Design review of the part built by this model. Coordinates are the model's own, in mm. A direction names the side the tool comes from. Coordinates: 2 decimals unless noted, no trailing zeros. Loops run counter-clockwise (first coordinate to the right, second up) from the corner with the lowest first, then second, coordinate; pieces in that order, holes last. Notation, with made-up numbers: (14, -3) -> (34, -3) arc R36 cw to (34, 36) -> close; hole circle Ø3 at (83.5, 62). An arc over 180 degrees is marked (long way). Use a Markdown table: item, result. Add a question column.
Q1. Take a section at A-A on y = 28. Write out the cut boundary in (x, z), plus the area to 3 significant figures.
Q2. Draft analysis for pull direction X (two halves, no side actions). For faces 3 (the face through (-107.984, 12, -49)), 4 (the face through (-17, 12, 39.984)), 5 (the face through (24, 5, -92)), state which applies: pulls with the +X half, pulls with the -X half, needs draft (parallel to the pull), parting line crosses it, or undercut.
Q3. Take a section at C-C on z = 25. Write out the cut boundary in (x, y), plus the area to 3 significant figures.
Q4. For probe 1 along Z at (x, y) = (-18.5, 8); probe 2 along Y at (x, z) = (-91, -137.5); probe 3 along Z at (x, y) = (69, 11), list the stretches that pass through material, from the lowest coordinate up.
Q5. Clearance check with flat-ended pins moving along their axes: pin 1 Ø10 at (x, y) = (23.5, 31) entering from +Z; pin 2 Ø8 at (y, z) = (43.5, -14) entering from +X; pin 3 Ø3 at (y, z) = (34, -48.5) entering from -X. State where each tip first meets the part, or that it passes through.
Q6. Take a section at B-B on z = -148.5. Write out the cut boundary in (x, y), plus the area to 3 significant figures.
Q7. For faces 1 (the face through (-42.558, 6.504, -135.362)), 2 (the face through (-88, 12, -150)), list the 3-axis set-ups (+Z, -Z, +X, -X, +Y, -Y) from which the entire face can be reached by the end or side of a thin tool; tool diameter is ignored.
from build123d import *

# Parameters (mm, degrees)
F1_DEPTH = 50
F2_DEPTH = 25
F4_DEPTH = 5
F5_R     = 5


with BuildPart() as f1:
    # F0 (on Front) → F1 (new body)
    with BuildSketch(Plane.XZ):
        with BuildLine():
            Line((-14.1471050896, 14.137164411), (-81.6470713128, -53.4102650408))
            ThreePointArc((-81.6470713128, -53.4102650408), (-81.4172585272, -82.8327909518), (-52.1131197981, -80.1860385553))
            Line((-52.1131197981, -80.1860385553), (14.1195211891, -14.1647139537))
            ThreePointArc((14.1195211891, -14.1647139537), (14.1509459034, 14.133319852), (-14.1471050896, 14.137164411))
        make_face()
        with BuildLine():
            ThreePointArc((-7.0735915388, 7.0685431839), (7.0736510846, 7.068483595), (7.0633719628, -7.0787552942))
            Line((7.0633719628, -7.0787552942), (-62.1351958298, -76.1269429069))
            ThreePointArc((-62.1351958298, -76.1269429069), (-75.7541474378, -74.3104584003), (-74.7048583437, -60.6110258843))
            Line((-74.7048583437, -60.6110258843), (-7.0735915388, 7.0685431839))
        make_face(mode=Mode.SUBTRACT)
    extrude(amount=-F1_DEPTH)

    # F0 (on Front) → F2 (join)
    with BuildSketch(Plane.XZ):
        with BuildLine():
            Line((102.0160578582, -0.0157058509), (62.0160578582, 39.9842941491))
            Line((62.0160578582, 39.9842941491), (-97.9839421418, 39.9842941491))
            ThreePointArc((-97.9839421418, 39.9842941491), (-105.0550099537, 37.055361961), (-107.9839421418, 29.9842941491))
            Line((-107.9839421418, 29.9842941491), (-107.9839421418, -130.0157058509))
            Line((-107.9839421418, -130.0157058509), (-67.9839421418, -170.0157058509))
            Line((-67.9839421418, -170.0157058509), (92.0160578582, -170.0157058509))
            ThreePointArc((92.0160578582, -170.0157058509), (99.0871256701, -167.0867736627), (102.0160578582, -160.0157058509))
            Line((102.0160578582, -160.0157058509), (102.0160578582, -0.0157058509))
        make_face()
        with BuildLine():
            ThreePointArc((93.0160578582, -91.0157058509), (90.0871256701, -98.0867736627), (83.0160578582, -101.0157058509))
            Line((83.0160578582, -101.0157058509), (57.0160578582, -101.0157058509))
            ThreePointArc((57.0160578582, -101.0157058509), (40.0454951097, -108.0451431024), (33.0160578582, -125.0157058509))
            Line((33.0160578582, -125.0157058509), (33.0160578582, -151.0157058509))
            ThreePointArc((33.0160578582, -151.0157058509), (30.0871256701, -158.0867736627), (23.0160578582, -161.0157058509))
            Line((23.0160578582, -161.0157058509), (-33.9839421418, -161.0157058509))
            ThreePointArc((-33.9839421418, -161.0157058509), (-41.0550099537, -158.0867736627), (-43.9839421418, -151.0157058509))
            Line((-43.9839421418, -151.0157058509), (-43.9839421418, -119.263347337))
            ThreePointArc((-43.9839421418, -119.263347337), (-41.9657763558, -113.2392023702), (-36.7258776257, -109.6466020559))
            ThreePointArc((-36.7258776257, -109.6466020559), (12.6262309135, -80.6258789061), (41.6469540632, -31.273770367))
            ThreePointArc((41.6469540632, -31.273770367), (45.2395543775, -26.0338716369), (51.2636993443, -24.0157058509))
            Line((51.2636993443, -24.0157058509), (83.0160578582, -24.0157058509))
            ThreePointArc((83.0160578582, -24.0157058509), (90.0871256701, -26.944638039), (93.0160578582, -34.0157058509))
            Line((93.0160578582, -34.0157058509), (93.0160578582, -91.0157058509))
        make_face(mode=Mode.SUBTRACT)
        with BuildLine():
            ThreePointArc((-52.1131197981, -80.1860385553), (-81.4172585272, -82.8327909518), (-81.6470713128, -53.4102650408))
            Line((-81.6470713128, -53.4102650408), (-14.1471050896, 14.137164411))
            ThreePointArc((-14.1471050896, 14.137164411), (14.1509459034, 14.133319852), (14.1195211891, -14.1647139537))
            Line((14.1195211891, -14.1647139537), (-52.1131197981, -80.1860385553))
        make_face(mode=Mode.SUBTRACT)
    extrude(amount=-F2_DEPTH)

    # F3 (on face) → F4 (join)
    with BuildSketch(Plane.XZ):
        with BuildLine():
            ThreePointArc((51.2636993443, -24.0157058509), (45.2395543775, -26.0338716369), (41.6469540632, -31.273770367))
            ThreePointArc((41.6469540632, -31.273770367), (12.6262309135, -80.6258789061), (-36.7258776257, -109.6466020559))
            ThreePointArc((-36.7258776257, -109.6466020559), (-41.9657763558, -113.2392023702), (-43.9839421418, -119.263347337))
            Line((-43.9839421418, -119.263347337), (-43.9839421418, -151.0157058509))
            ThreePointArc((-43.9839421418, -151.0157058509), (-41.0550099537, -158.0867736627), (-33.9839421418, -161.0157058509))
            Line((-33.9839421418, -161.0157058509), (23.0160578582, -161.0157058509))
            ThreePointArc((23.0160578582, -161.0157058509), (30.0871256701, -158.0867736627), (33.0160578582, -151.0157058509))
            Line((33.0160578582, -151.0157058509), (33.0160578582, -125.0157058509))
            ThreePointArc((33.0160578582, -125.0157058509), (40.0454951097, -108.0451431024), (57.0160578582, -101.0157058509))
            Line((57.0160578582, -101.0157058509), (83.0160578582, -101.0157058509))
            ThreePointArc((83.0160578582, -101.0157058509), (90.0871256701, -98.0867736627), (93.0160578582, -91.0157058509))
            Line((93.0160578582, -91.0157058509), (93.0160578582, -34.0157058509))
            ThreePointArc((93.0160578582, -34.0157058509), (90.0871256701, -26.944638039), (83.0160578582, -24.0157058509))
            Line((83.0160578582, -24.0157058509), (51.2636993443, -24.0157058509))
        make_face()
    extrude(amount=-F4_DEPTH)

    # F5
    f5_edges = [f1.edges().sort_by_distance(p)[0] for p in [
        (67.139879, 5, -24.015706),
        (83.016058, 15, -24.015706),
        (67.139879, 25, -24.015706),
        (51.263699, 15, -24.015706),
        (45.239554, 5, -26.033872),
        (12.626231, 5, -80.625879),
        (-41.965776, 5, -113.239202),
        (-43.983942, 5, -135.139527),
        (-41.05501, 5, -158.086774),
        (-5.483942, 5, -161.015706),
        (30.087126, 5, -158.086774),
        (33.016058, 5, -138.015706),
        (40.045495, 5, -108.045143),
        (70.016058, 5, -101.015706),
        (90.087126, 5, -98.086774),
        (93.016058, 5, -62.515706),
        (90.087126, 5, -26.944638),
    ]]
    fillet(f5_edges, radius=F5_R)


solid = f1.part
Answer list:
| question | item | result |
|---|---|---|
| 1 | outline | (-81.65, -53.41) arc R20 ccw (long way) to (-52.11, -80.19) -> (14.12, -14.16) arc R20 ccw to (-14.15, 14.14) -> close; hole (-74.7, -60.61) arc R10 ccw to (-62.14, -76.13) -> (7.06, -7.08) arc R10 ccw to (-7.07, 7.07) -> close |
| 1 | area | 2,860 mm² |
| 2 | face 3 | pulls with the -X half |
| 2 | face 4 | needs draft |
| 2 | face 5 | undercut |
| 3 | outline | (-107.98, 0) -> (77, 0) -> (77, 25) -> (-107.98, 25) -> close |
| 3 | area | 4,620 mm² |
| 4 | probe 1 | -170.02 to -160.6, -103.18 to -32.59, -4.37 to 39.98 |
| 4 | probe 2 | 0 to 25 |
| 4 | probe 3 | -170.02 to -101.02, -24.02 to 33 |
| 5 | pin 1 | z = 7.6 |
| 5 | pin 2 | x = 17.32 |
| 5 | pin 3 | x = -78.24 |
| 6 | outline | (-89.5, 0) -> (102.02, 0) -> (102.02, 25) -> (38.02, 25) arc R5 ccw to (33.02, 20) -> (33.02, 10) arc R5 cw to (28.02, 5) -> (-38.98, 5) arc R5 cw to (-43.98, 10) -> (-43.98, 20) arc R5 ccw to (-48.98, 25) -> (-89.5, 25) -> close |
| 6 | area | 3,250 mm² |
| 7 | face 1 | +Y |
| 7 | face 2 | -Z, -X, +Y, -Y |
